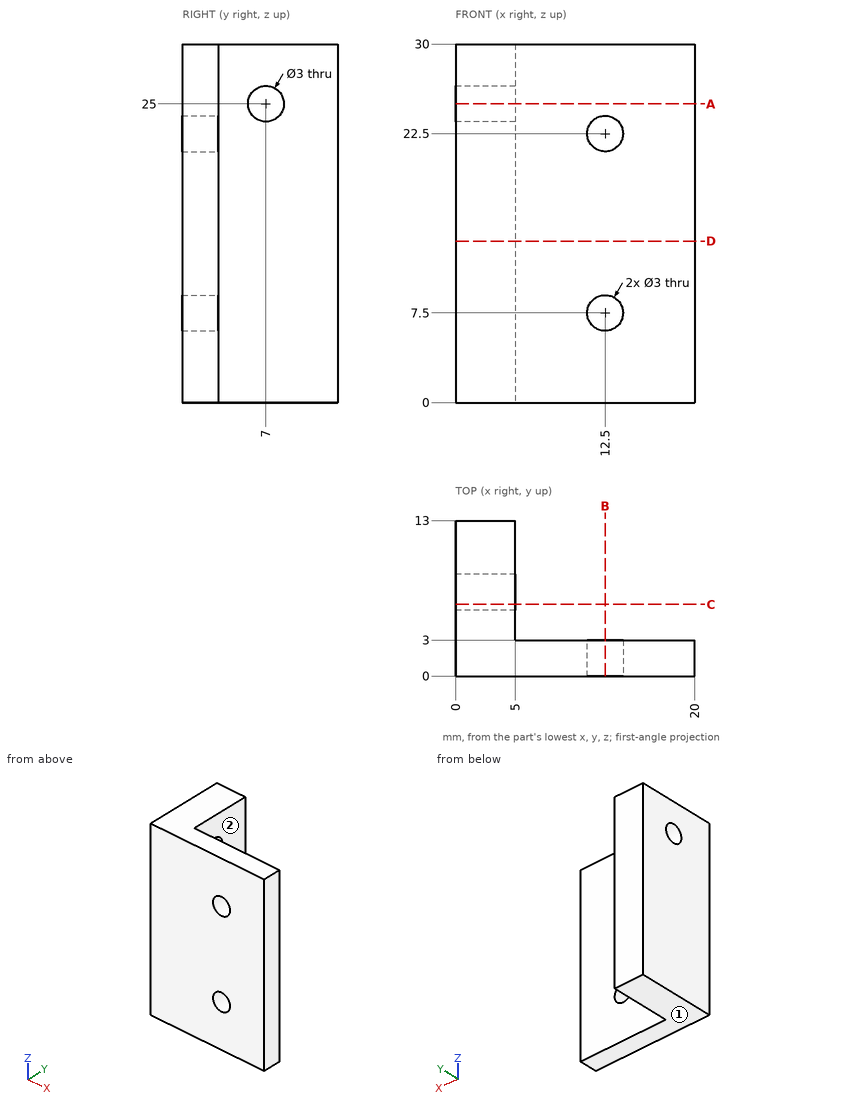
Source: three-view drawing plus pictorial views. Frame: mm from the lowest corner of the part. A direction names the side the tool comes from. Give positions to 0.01 mm unless a question says otherwise; leave off trailing zeros. Order: outer loops, then holes, each group sorted by start corner. A loop starts at its lowest first (then second) coordinate and runs counter-clockwise, first axis right, second up. Notation, with made-up numbers: (56.5, 6.25) - (109.5, 6.25) arc R29 cw to (109.5, 34.25) - close; hole circle Ø1 at (0.5, -22). An arc over 180 degrees is marked (long way). Put each result on its own line as item: value.
Item 1: Section query C-C, the plane y = 6. Return loops of the section in (x, z), then the cut area to 3 significant figures.
Found:
outline: (0, 0) - (5, 0) - (5, 23.88) - (0, 23.88) - close; (0, 26.12) - (5, 26.12) - (5, 30) - (0, 30) - close
area: 139 mm^2
Item 2: Section query A-A, the plane z = 25. Return loops of the section in (x, y), then the cut area to 3 significant figures.
Found:
outline: (0, 0) - (20, 0) - (20, 3) - (5, 3) - (5, 5.5) - (0, 5.5) - close; (0, 8.5) - (5, 8.5) - (5, 13) - (0, 13) - close
area: 95.0 mm^2
Item 3: Ray query, L1, parallel to Z at x = 12.5, y = 1.9; L2, parallel to X at y = 1.1, z = 7.5; L3, parallel to Y at x = 1.8, z = 25. Return the intervals inside material, ascending. Write a range as from..to.
Found:
L1: z = 0..6, 9..21, 24..30
L2: x = 0..11, 14..20
L3: y = 0..5.5, 8.5..13
Item 4: Section query D-D, the plane z = 13.5. Return loops of the section in (x, y), then the cut area to 3 significant figures.
Found:
outline: (0, 0) - (20, 0) - (20, 3) - (5, 3) - (5, 13) - (0, 13) - close
area: 110 mm^2
Item 5: Contact query for flat-ended pins moving along their axis: pin 1 (1.5 mm diameter, centred on y = 10.5, z = 20, fed in from +X); pin 2 (4.5 mm diameter, centred on x = 16, z = 8.5, fed in from +Y). Output: stop coordinate, or through.
Found:
pin 1: stops at x = 5
pin 2: stops at y = 3
Item 6: Access query for the marked faces 1 and 2. Directions: +Z, -Z, +X, -X, +Y, -Y. A direction counts if a zero-diameter tool reaches every point of the face in a straight line with its end or side. Return the directions, or none.
Found:
face 1: -Z, +X, -X, +Y, -Y
face 2: +Z, -Z, +X, +Y
Item 7: Section query B-B, the plane x = 12.5. Return loops of the section in (y, z), then the cut area to 3 significant figures.
Found:
outline: (0, 0) - (3, 0) - (3, 6) - (0, 6) - close; (0, 9) - (3, 9) - (3, 21) - (0, 21) - close; (0, 24) - (3, 24) - (3, 30) - (0, 30) - close
area: 72.0 mm^2
